from build123d import *

# Parameters (mm, degrees)
BOSS_EXTRUDE1_DEPTH = 9
SKETCH2_W           = 5
SKETCH2_H           = 9
CUT_EXTRUDE1_DEPTH  = 3
BOSS_EXTRUDE2_DEPTH = 3
SKETCH4_W           = 4
SKETCH4_H           = 4
BOSS_EXTRUDE3_DEPTH = 4.5


with BuildPart() as part:
    # Sketch1 → Boss-Extrude1 (new body)
    with BuildSketch(Plane.XY):
        with BuildLine():
            Line((3, 0), (3, -4))
            Line((3, -4), (5, -4))
            Line((5, -4), (5, 0))
            ThreePointArc((5, 0), (0, 5), (-5, 0))
            Line((-5, 0), (-5, -4))
            Line((-5, -4), (-3, -4))
            Line((-3, -4), (-3, 0))
            ThreePointArc((-3, 0), (0, 3), (3, 0))
        make_face()
    extrude(amount=BOSS_EXTRUDE1_DEPTH)

    # Sketch2 → Cut-Extrude1 (cut)
    with BuildSketch(Plane.XY.offset(9)):
        with Locations((2.5, 0.5)):
            Rectangle(SKETCH2_W, SKETCH2_H)
    extrude(amount=-CUT_EXTRUDE1_DEPTH, mode=Mode.SUBTRACT)



with BuildPart() as body_2:
    # Sketch3 → Boss-Extrude2 (new body)
    with BuildSketch(Plane(origin=(0, 0, 0), x_dir=(-1, 0, 0), z_dir=(0, 0, -1))):
        with BuildLine():
            Line((-5, -4), (-7, -4))
            Line((-7, -4), (-7, 0))
            Line((-7, 0), (-4, 3))
            ThreePointArc((-4, 3), (-4.74341649, 1.58113883), (-5, 0))
            Line((-5, 0), (-5, -4))
        make_face()
    extrude(amount=-BOSS_EXTRUDE2_DEPTH)


with BuildPart() as part_1:
    add(part.part)

    add(body_2.part)  # Boss-Extrude3 merges body 2
    # Sketch4 → Boss-Extrude3 (add)
    with BuildSketch(Plane.XY.offset(3)):
        with Locations((5, -2)):
            Rectangle(SKETCH4_W, SKETCH4_H)
    extrude(amount=BOSS_EXTRUDE3_DEPTH)


solid = part_1.part
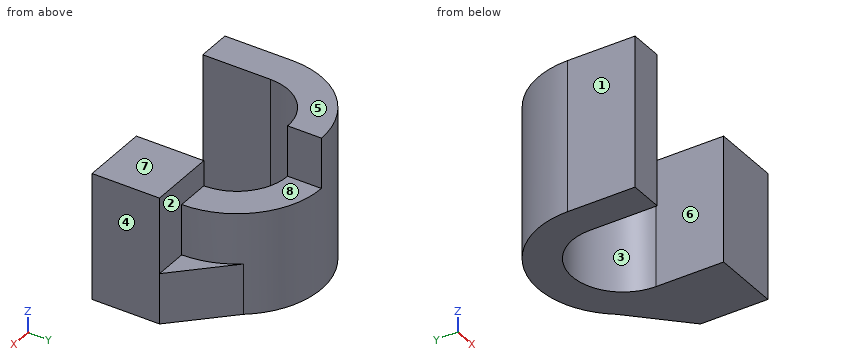
Input: part model. Units: mm. Frame: model coordinates. Face numbers are marked on the shaded views. A direction names the side the tool comes from. Give positions to 0.01 mm unless a question says otherwise; leave off trailing zeros. Loops run counter-clockwise (first coordinate to the right, second up) from the corner with the lowest first, then second, coordinate; pieces in that order, holes last. Notation, with made-up numbers: (40, 6.5) -> (86, 6.5) arc R10 cw to (86, 18.5) -> close; hole circle Ø6 at (19.25, 27.5). An arc over 180 degrees is marked (long way). Answer as a JSON object with one key per item and string values. Group by question number.
Item 1: Pull-direction query (X, two-part tool) for the marked faces 1, 2, 3 and 4; classes: released by +X, released by -X, zero draft, split by the parting line, or undercut.
Item 2: Cut plane D-D, the plane x = 3.75. Return the cut outline in (y, z).
Item 3: Reachability of the marked faces 5, 6, 7 and 8 from +Z, -Z, +X, -X, +Y, -Y: full face, straight path, thin tool, end or side. Return the list, or none.
Item 4: Cut plane A-A, the plane y = -1.75. Return the cut outline in (x, z), and give its area (3 significant figures).
Item 5: Pin query (flat end, axial travel): P1, Ø1, axis at y = 4, z = 7.5, coming from the +X side; P2, Ø2, axis at x = 5, z = 6, coming from the +Y side; P3, Ø1.2, axis at x = 5.5, y = -2.5, coming from the +Z side. Return the tip coordinate at first contact, or that it passes through.
Item 6: Cut plane C-C, the plane z = 5.75. Return the cut outline in (x, y), and give its area (3 significant figures).
Item 7: Cut plane B-B, the plane z = 2. Return the cut outline in (x, y), and give its area (3 significant figures).
Item 8: Line query: probe 1 along X at (y, z) = (-0.5, 2.5); probe 2 along Z at (x, y) = (4.25, 1.75); probe 3 along Y at (x, z) = (-4, 7). Output: solid intervals per line, ascending.
Checks:
{
 "1": {"face 1": "released by -X", "face 2": "zero draft", "face 3": "undercut", "face 4": "released by +X"},
 "2": {"outline": "(-4, 0) -> (3.31, 0) -> (3.31, 6) -> (0, 6) -> (0, 7.5) -> (-4, 7.5) -> close"},
 "3": {"face 5": "+Z, +X, -X, +Y, -Y", "face 6": "+Z, -Z, -Y", "face 7": "+Z, +X, +Y, -Y", "face 8": "+Z, +X, +Y"},
 "4": {"outline": "(-5, 0) -> (-3, 0) -> (-3, 9) -> (-5, 9) -> close; (3, 0) -> (7, 0) -> (7, 7.5) -> (3, 7.5) -> close", "area": "48.0 mm²"},
 "5": {"P1": "stops at x = 0", "P2": "stops at y = 3", "P3": "stops at z = 7.5"},
 "6": {"outline": "(-5, -4) -> (-3, -4) -> (-3, 0) arc R3 cw to (3, 0) -> (3, -4) -> (7, -4) -> (7, 0) -> (5, 0) arc R5 ccw to (-5, 0) -> close", "area": "49.1 mm²"},
 "7": {"outline": "(-5, -4) -> (-3, -4) -> (-3, 0) arc R3 cw to (3, 0) -> (3, -4) -> (7, -4) -> (7, 0) -> (4, 3) arc R5 ccw to (-5, 0) -> close", "area": "51.6 mm²"},
 "8": {"probe 1": "x = -5 to -3, 3 to 7", "probe 2": "z = 0 to 6", "probe 3": "y = -4 to 3"}
}
